For this review, take the finished solid that the model builds, in its own axes (mm). A direction names the side the tool comes from. Coordinates: 2 decimals unless noted, no trailing zeros. Loops run counter-clockwise (first coordinate to the right, second up) from the corner with the lowest first, then second, coordinate; pieces in that order, holes last. Notation, with made-up numbers: M 17,14 L 25,14 A11 cw 25,18 Z; hole C -29.75,43 d1. An arc over 180 degrees is marked long. Put each result on its own line as item: value.
```python
from build123d import *

# Parameters (mm, degrees)
ESQUISSE3_R      = 2
ESQUISSE3_R_2    = 10
EXTRUSION2_DEPTH = 19


with BuildPart() as part:
    # Esquisse1 → Révolution1 (revolve)
    with BuildSketch(Plane.XY):
        Polygon((-6.5, 17), (-6.5, 41), (-8.5, 41), (-8.5, 19), (-11, 19), (-11, -3), (-10, -3), (-10, 17), align=None)
    revolve(axis=Axis((0, 0, 0), (0, 1, 0)))

    # Esquisse3 → Extrusion2 (add)
    with BuildSketch(Plane(origin=(0, 19, 0), x_dir=(1, 0, 0), z_dir=(0, 1, 0))):
        with BuildLine():
            Line((-12.449899598, -13), (-7.924146363, -13))
            Line((-7.924146363, -13), (-6.438678833, -8.918711504))
            ThreePointArc((-6.438678833, -8.918711504), (0, -11), (6.438678833, -8.918711504))
            Line((6.438678833, -8.918711504), (7.924146363, -13))
            Line((7.924146363, -13), (12.449899598, -13))
            ThreePointArc((12.449899598, -13), (12.727922061, -12.727922061), (13, -12.449899598))
            Line((13, -12.449899598), (13, -7.924146363))
            Line((13, -7.924146363), (8.918711504, -6.438678833))
            ThreePointArc((8.918711504, -6.438678833), (11, 0), (8.918711504, 6.438678833))
            Line((8.918711504, 6.438678833), (13, 7.924146363))
            Line((13, 7.924146363), (13, 12.449899598))
            ThreePointArc((13, 12.449899598), (12.727922061, 12.727922061), (12.449899598, 13))
            Line((12.449899598, 13), (7.924146363, 13))
            Line((7.924146363, 13), (6.438678833, 8.918711504))
            ThreePointArc((6.438678833, 8.918711504), (0, 11), (-6.438678833, 8.918711504))
            Line((-6.438678833, 8.918711504), (-7.924146363, 13))
            Line((-7.924146363, 13), (-12.449899598, 13))
            ThreePointArc((-12.449899598, 13), (-12.727922061, 12.727922061), (-13, 12.449899598))
            Line((-13, 12.449899598), (-13, 7.924146363))
            Line((-13, 7.924146363), (-8.918711504, 6.438678833))
            ThreePointArc((-8.918711504, 6.438678833), (-11, 0), (-8.918711504, -6.438678833))
            Line((-8.918711504, -6.438678833), (-13, -7.924146363))
            Line((-13, -7.924146363), (-13, -12.449899598))
            ThreePointArc((-13, -12.449899598), (-12.727922061, -12.727922061), (-12.449899598, -13))
        make_face()
        with Locations((10.606601718, 10.606601718)):
            Circle(ESQUISSE3_R, mode=Mode.SUBTRACT)
        with Locations((-10.606601718, -10.606601718)):
            Circle(ESQUISSE3_R, mode=Mode.SUBTRACT)
        with Locations((-10.606601718, 10.606601718)):
            Circle(ESQUISSE3_R, mode=Mode.SUBTRACT)
        with Locations((10.606601718, -10.606601718)):
            Circle(ESQUISSE3_R, mode=Mode.SUBTRACT)
        Circle(ESQUISSE3_R_2, mode=Mode.SUBTRACT)
    extrude(amount=-EXTRUSION2_DEPTH)


solid = part.part
```
(1) Add section C-C (y = 34). Write out the cut boundary in (x, z).
Determined:
outline: C 0,0 d17; hole C 0,0 d13
(2) Add section A-A (x = 0). Write out the cut boundary in (y, z).
Determined:
outline: M -3,-11 L 19,-11 L 19,-8.5 L 41,-8.5 L 41,-6.5 L 17,-6.5 L 17,-10 L -3,-10 Z; M -3,10 L 17,10 L 17,6.5 L 41,6.5 L 41,8.5 L 19,8.5 L 19,11 L -3,11 Z
(3) Tool access review of faces 1 (the flat face through (9, 19, 0)), 2 (the flat face through (-9, 0, 9)), 3 (the flat face through (9, 0, -9)), 4 (the flat face through (10.93, 9.63, -7.17)): name each direction out of +Z, -Z, +X, -X, +Y, -Y from which nothing blocks a thin tool from reaching the whole face with its end or side.
Determined:
face 1: +Y
face 2: +Z, -X, -Y
face 3: -Z, +X, -Y
face 4: +X, +Y, -Y
(4) For pin 1 (2 mm diameter, centred on x = -9.5, z = 10.5, fed in from -Y); pin 2 (6.5 mm diameter, centred on x = 10.61, z = 10.61, fed in from +Y); pin 3 (3 mm diameter, centred on x = -10.61, z = -10.61, fed in from -Y); pin 4 (10 mm diameter, centred on x = -2, z = 4.5, fed in from -Y), all flat-tipped, find the tip position at first contact; note any pin that passes through.
Determined:
pin 1: stops at y = 0
pin 2: stops at y = 19
pin 3: passes through
pin 4: stops at y = 17
(5) Add section D-D (x = 10.5). Write out the cut boundary in (y, z), plus the area to 3 significant figures.
Determined:
outline: M -3,-3.28 L 19,-3.28 L 19,3.28 L -3,3.28 Z; M 0,-13 L 19,-13 L 19,-12.6 L 0,-12.6 Z; M 0,-8.61 L 19,-8.61 L 19,-7.01 L 0,-7.01 Z; M 0,7.01 L 19,7.01 L 19,8.61 L 0,8.61 Z; M 0,12.6 L 19,12.6 L 19,13 L 0,13 Z
area: 220 mm^2
(6) Add section B-B (z = 4.25). Write out the cut boundary in (x, y), plus the area to 3 significant figures.
Determined:
outline: M -10.15,-3 L -9.05,-3 L -9.05,17 L -4.92,17 L -4.92,41 L -7.36,41 L -7.36,19 L -10.15,19 Z; M 4.92,17 L 9.05,17 L 9.05,-3 L 10.15,-3 L 10.15,19 L 7.36,19 L 7.36,41 L 4.92,41 Z
area: 172 mm^2
(7) Draft analysis for pull direction Z (two halves, no side actions). For faces 5 (the flat face through (-13, 10, -10)), 6 (the flat face through (-10.93, 9.63, 7.17)), 7 (the flat face through (7.17, 9.63, 10.93)), state which applies: +Z half, -Z half, draft (parallel to the pull), parting line (faces both ways), or undercut.
Determined:
face 5: draft
face 6: undercut
face 7: +Z half
(8) Wall thickness on line 1 along X through (y, z) = (-2.25, 0); line 2 along X through (y, z) = (9, -9.25); line 3 along Y through (x, z) = (-7, -7.5): over which ranges is each line inside the solid? List them lowest first. Write a range as [from, to].
Determined:
line 1: x = [-11, -10], [10, 11]
line 2: x = [-13, -12.08], [-9.14, -6.56], [-5.95, -3.8], [3.8, 5.95], [6.56, 9.14], [12.08, 13]
line 3: y = [-3, 19]
